```python
from build123d import *

# Parameters (mm, degrees)
SKETCH1_W           = 530
SKETCH1_H           = 475
BOSS_EXTRUDE1_DEPTH = 11
SKETCH2_W           = 306
SKETCH2_H           = 286
BOSS_EXTRUDE2_DEPTH = 12
SKETCH3_R           = 10
SKETCH3_R_2         = 9
CUT_EXTRUDE1_DEPTH  = 357.532256605
SKETCH4_R           = 18
CUT_EXTRUDE2_DEPTH  = 358.473425586
SKETCH5_R           = 32.5
CUT_EXTRUDE3_DEPTH  = 14
FILLET1_R           = 10


with BuildPart() as part:
    # Sketch1 → Boss-Extrude1 (new, symmetric)
    with BuildSketch(Plane(origin=(0, 0, 0), x_dir=(1, 0, 0), z_dir=(0, 1, 0))):
        Rectangle(SKETCH1_W, SKETCH1_H)
    extrude(amount=BOSS_EXTRUDE1_DEPTH, both=True)

    # Sketch2 → Boss-Extrude2 (add)
    with BuildSketch(Plane(origin=(0, 11, 0), x_dir=(1, 0, 0), z_dir=(0, 1, 0))):
        Rectangle(SKETCH2_W, SKETCH2_H)
    extrude(amount=BOSS_EXTRUDE2_DEPTH)

    # Sketch3 → Cut-Extrude1 (cut, through all)
    with BuildSketch(Plane(origin=(0, 11, 0), x_dir=(1, 0, 0), z_dir=(0, 1, 0))):
        with Locations(Location((-245, 217.5, 0), (0, 0, 270))):
            Circle(SKETCH3_R)
        with Locations(Location((-120, 217.5, 0), (0, 0, 270))):
            Circle(SKETCH3_R_2)
        with Locations(Location((-245, 110, 0), (0, 0, 270))):
            Circle(SKETCH3_R_2)
        with Locations(Location((120, 217.5, 0), (0, 0, 90))):
            Circle(SKETCH3_R_2)
        with Locations(Location((245, 217.5, 0), (0, 0, 90))):
            Circle(SKETCH3_R)
        with Locations(Location((245, 110, 0), (0, 0, 90))):
            Circle(SKETCH3_R_2)
        with Locations(Location((245, -110, 0), (0, 0, 270))):
            Circle(SKETCH3_R_2)
        with Locations(Location((245, -217.5, 0), (0, 0, 270))):
            Circle(SKETCH3_R)
        with Locations(Location((120, -217.5, 0), (0, 0, 270))):
            Circle(SKETCH3_R_2)
        with Locations(Location((-120, -217.5, 0), (0, 0, 90))):
            Circle(SKETCH3_R_2)
        with Locations(Location((-245, -110, 0), (0, 0, 90))):
            Circle(SKETCH3_R_2)
        with Locations(Location((-245, -217.5, 0), (0, 0, 90))):
            Circle(SKETCH3_R)
    extrude(amount=-CUT_EXTRUDE1_DEPTH, mode=Mode.SUBTRACT)

    # Sketch4 → Cut-Extrude2 (cut, through all)
    with BuildSketch(Plane(origin=(0, 23, 0), x_dir=(1, 0, 0), z_dir=(0, 1, 0))):
        with Locations(Location((57, 93, 0), (0, 0, 270))):
            Circle(SKETCH4_R)
    extrude(amount=-CUT_EXTRUDE2_DEPTH, mode=Mode.SUBTRACT)

    # Sketch5 → Cut-Extrude3 (cut)
    with BuildSketch(Plane.XZ.offset(11)):
        with Locations(Location((57, -93, 0), (0, 0, 270))):
            Circle(SKETCH5_R)
    extrude(amount=-CUT_EXTRUDE3_DEPTH, mode=Mode.SUBTRACT)

    # Fillet1
    fillet1_edges = [part.edges().sort_by_distance(p)[0] for p in [
        (153, 17, 143),
        (153, 17, -143),
        (-153, 17, -143),
        (-153, 17, 143),
        (265, 0, 237.5),
        (-265, 0, 237.5),
        (-265, 0, -237.5),
        (265, 0, -237.5),
    ]]
    fillet(fillet1_edges, radius=FILLET1_R)


solid = part.part
```
Read the model definition and answer for the solid it produces. Units are mm, in the model's axes. A direction names the side the tool comes from. Coordinates: 2 decimals unless noted, no trailing zeros. Write each loop counter-clockwise with the first axis right and the second up, starting at its lowest first coordinate (ties: lowest second). Pieces come first, ordered by that corner, then holes. Notation, with made-up numbers: (31, 10) - (59, 10) arc R21 ccw to (59, 32) - close; hole circle Ø1 at (54.25, 18.25). An arc over 180 degrees is marked (long way). Answer as a JSON object with one key per item and string values. Group by question number.
1. A cutting plane is placed at A-A (x = 120). Determine the outline of the cut face in (y, z).
2. A cutting plane is placed at C-C (x = 245). Determine the outline of the cut face in (y, z), plus the area to 3 significant figures.
3. A cutting plane is placed at B-B (z = -217.5). Determine the outline of the cut face in (x, y), plus the area to 3 significant figures.
4. Consider L1, parallel to X at y = -5, z = -217.5; L2, parallel to X at y = -6, z = -111; L3, parallel to X at y = 1, z = -110. Determine where each line is inside the solid, lowest interval first. Write a range as [from, to].
5. The mould has two halves that part along X. Classify faces 1 (the flat face through (-153, 17, 2)), 2 (the cylindrical face through (-237.015, 0.154, 105.847)), 3 (the cylindrical face through (252.985, 0.154, -114.153)), 4 (the flat face through (-2, 17, 143)): +X half, -X half, draft (parallel to the pull), parting line (faces both ways), or undercut.
6. Which of the six approach directions +Z, -Z, +X, -X, +Y, -Y give full straight-line access (tool end or side, diameter ignored) to faces 5 (the flat face through (-4, 11, 155)), 6 (the cylindrical face through (-120.4, 0.15, 226.49)), 7 (the flat face through (153, 17, 2))?
7. Each of these flat-tipped pins is pushed along its axis until it touches: P1, Ø9.5, axis at x = -36, y = 16, coming from the -Z side; P2, Ø16, axis at x = -245, z = -110, coming from the -Y side; P3, Ø23.5, axis at x = 120, z = 217.5, coming from the +Y side; P4, Ø5, axis at x = -48.5, y = 17, coming from the +Z side. Where does it stop, or does it pass through?
8. A cutting plane is placed at D-D (z = 27.5). Determine the outline of the cut face in (x, y).
Worked out:
{
 "1": {"outline": "(-11, -237.5) - (11, -237.5) - (11, -226.5) - (-11, -226.5) - close; (-11, -208.5) - (11, -208.5) - (11, -143) - (23, -143) - (23, 143) - (11, 143) - (11, 208.5) - (-11, 208.5) - close; (-11, 226.5) - (11, 226.5) - (11, 237.5) - (-11, 237.5) - close"},
 "2": {"outline": "(-11, -237.5) - (11, -237.5) - (11, -227.5) - (-11, -227.5) - close; (-11, -207.5) - (11, -207.5) - (11, -119) - (-11, -119) - close; (-11, -101) - (11, -101) - (11, 101) - (-11, 101) - close; (-11, 119) - (11, 119) - (11, 207.5) - (-11, 207.5) - close; (-11, 227.5) - (11, 227.5) - (11, 237.5) - (-11, 237.5) - close", "area": "8,780 mm²"},
 "3": {"outline": "(-265, -11) - (-255, -11) - (-255, 11) - (-265, 11) - close; (-235, -11) - (-129, -11) - (-129, 11) - (-235, 11) - close; (-111, -11) - (111, -11) - (111, 11) - (-111, 11) - close; (129, -11) - (235, -11) - (235, 11) - (129, 11) - close; (255, -11) - (265, -11) - (265, 11) - (255, 11) - close", "area": "9,990 mm²"},
 "4": {"L1": "x = [-265, -255], [-235, -129], [-111, 111], [129, 235], [255, 265]", "L2": "x = [-265, -253.94], [-236.06, 29.94], [84.06, 236.06], [253.94, 265]", "L3": "x = [-265, -254], [-236, 29.3], [84.7, 236], [254, 265]"},
 "5": {"face 1": "-X half", "face 2": "undercut", "face 3": "undercut", "face 4": "draft"},
 "6": {"face 5": "+Y", "face 6": "+Y, -Y", "face 7": "+Z, -Z, +X, +Y"},
 "7": {"P1": "stops at z = -143", "P2": "passes through", "P3": "stops at y = 11", "P4": "stops at z = 143"},
 "8": {"outline": "(-265, -11) - (265, -11) - (265, 11) - (153, 11) - (153, 23) - (-153, 23) - (-153, 11) - (-265, 11) - close"}
}
